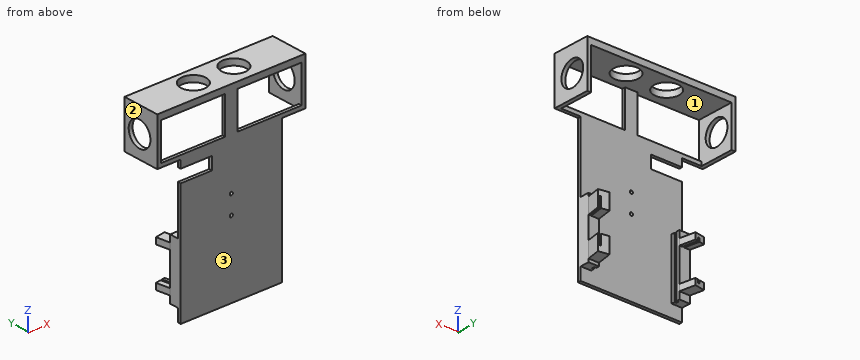
```python
from build123d import *

# Parameters (mm, degrees)
SKETCH1_W            = 95
SKETCH1_H            = 22
SKETCH1_R            = 8
BOSS_EXTRUDE1_DEPTH  = 4
SKETCH2_W            = 41
SKETCH2_H            = 23.5
BOSS_EXTRUDE2_DEPTH  = 2
BOSS_EXTRUDE3_START  = -70
BOSS_EXTRUDE3_DEPTH  = 38
BOSS_EXTRUDE5_DEPTH  = 10
BOSS_EXTRUDE6_DEPTH  = 10
SKETCH10_R           = 1
CUT_EXTRUDE1_DEPTH   = 4
BOSS_EXTRUDE11_START = 45
SKETCH11_W           = 30
SKETCH11_H           = 24
SKETCH11_R           = 8
BOSS_EXTRUDE11_DEPTH = 2.5
BOSS_EXTRUDE12_START = -47.5
SKETCH11_2_W         = 30
SKETCH11_2_H         = 24
SKETCH11_2_R         = 8
BOSS_EXTRUDE12_DEPTH = 2.5


with BuildPart() as part:
    # Sketch1 → Boss-Extrude1 (new body)
    with BuildSketch(Plane.XY):
        Rectangle(SKETCH1_W, SKETCH1_H)
        with Locations((-13, 0)):
            Circle(SKETCH1_R, mode=Mode.SUBTRACT)
        with Locations((13, 0)):
            Circle(SKETCH1_R, mode=Mode.SUBTRACT)
    extrude(amount=BOSS_EXTRUDE1_DEPTH)

    # Sketch2 → Boss-Extrude2 (add)
    with BuildSketch(Plane(origin=(0, -11, 0), x_dir=(-1, 0, 0), z_dir=(0, -1, 0))):
        Polygon((-32.5, 116), (32.5, 116), (32.5, 39), (12.5, 39), (12.5, 31), (32.5, 31), (32.5, 26), (47.5, 26), (47.5, -4), (32.5, -4), (-32.5, -4), (-47.5, -4), (-47.5, 26), (-32.5, 26), align=None)
        with Locations((-24.5, 11.75)):
            Rectangle(SKETCH2_W, SKETCH2_H, mode=Mode.SUBTRACT)
        with Locations((24.5, 11.75)):
            Rectangle(SKETCH2_W, SKETCH2_H, mode=Mode.SUBTRACT)
    extrude(amount=BOSS_EXTRUDE2_DEPTH)

    # Sketch4 → Boss-Extrude3 (add)
    with BuildSketch(Plane.XY.offset(BOSS_EXTRUDE3_START)):
        Polygon((-25.8, -11), (-25.8, -9), (-27, -9), (-27, -7.3), (-25.8, -7.3), (-25.8, -5.3), (-32.5, -5.3), (-32.5, -11), align=None)
        Polygon((32.5, -5.3), (32.5, -11), (25.8, -11), (25.8, -9), (27, -9), (27, -7.3), (25.8, -7.3), (25.8, -5.3), align=None)
    extrude(amount=-BOSS_EXTRUDE3_DEPTH)

    # Sketch7 → Boss-Extrude5 (add)
    with BuildSketch(Plane(origin=(0.128388188, -0.728125596, 0), x_dir=(0, 0, 1), z_dir=(-0.17364817766693402, 0.9848077530122075, 0))):
        Polygon((-74.5, -26.328375369), (-74.5, -32.926587315), (-78.5, -32.926587315), (-78.5, -29.426587315), (-76.5, -29.426587315), (-76.5, -28.226587315), (-78.5, -28.226587315), (-78.5, -26.328375369), align=None)
        Polygon((-101.5, -28.226587315), (-99.5, -28.226587315), (-99.5, -26.328375369), (-103.5, -26.328375369), (-103.5, -32.926587315), (-99.5, -32.926587315), (-99.5, -29.426587315), (-101.5, -29.426587315), align=None)
    extrude(amount=BOSS_EXTRUDE5_DEPTH)

    # Sketch8 → Boss-Extrude6 (add)
    with BuildSketch(Plane(origin=(-0.128388188, -0.728125596, 0), x_dir=(0, 0, 1), z_dir=(0.17364817766692736, 0.9848077530122086, 0))):
        Polygon((-82, 26.328375369), (-82, 31.176587315), (-75.5, 31.176587315), (-75.5, 32.226587315), (-82, 32.226587315), (-82, 32.926587315), (-72, 32.926587315), (-72, 26.328375369), align=None)
        Polygon((-96, 32.226587315), (-96, 32.926587315), (-106, 32.926587315), (-106, 26.328375369), (-96, 26.328375369), (-96, 31.176587315), (-102.5, 31.176587315), (-102.5, 32.226587315), align=None)
    extrude(amount=BOSS_EXTRUDE6_DEPTH)

    # Sketch10 → Cut-Extrude1 (cut)
    with BuildSketch(Plane.XZ.offset(13)):
        with Locations((0, -56)):
            Circle(SKETCH10_R)
        with Locations((0, -68)):
            Circle(SKETCH10_R)
    extrude(amount=-CUT_EXTRUDE1_DEPTH, mode=Mode.SUBTRACT)

    # Sketch11 → Boss-Extrude11 (add)
    with BuildSketch(Plane(origin=(0, 0, 0), x_dir=(0, 0, -1), z_dir=(1, 0, 0)).offset(BOSS_EXTRUDE11_START)):
        with Locations((11, -1)):
            Rectangle(SKETCH11_W, SKETCH11_H)
        with Locations((12, 0)):
            Circle(SKETCH11_R, mode=Mode.SUBTRACT)
    extrude(amount=BOSS_EXTRUDE11_DEPTH)

    # Sketch11<2> → Boss-Extrude12 (add)
    with BuildSketch(Plane(origin=(0, 0, 0), x_dir=(0, 0, -1), z_dir=(1, 0, 0)).offset(BOSS_EXTRUDE12_START)):
        with Locations((11, -1)):
            Rectangle(SKETCH11_2_W, SKETCH11_2_H)
        with Locations((12, 0)):
            Circle(SKETCH11_2_R, mode=Mode.SUBTRACT)
    extrude(amount=BOSS_EXTRUDE12_DEPTH)


solid = part.part
```
Source: CAD feature listing. Evaluate the final solid. Frame: model axes, mm. Face numbers are marked on the shaded views. Give positions to 0.01 mm unless a question says otherwise; leave off trailing zeros. Loops run counter-clockwise (first coordinate to the right, second up) from the corner with the lowest first, then second, coordinate; pieces in that order, holes last. Notation, with made-up numbers: (72, -32.75) - (78, -32.75) arc R35 cw to (78, 2.25) - close; hole circle Ø3 at (84, -18). An arc over 180 degrees is marked (long way). Use CSV: the item, a comma, the result in double quotes. Start each with the question number.
1. Draft query along X for the marked faces 1, 2 and 3. Return one class per face: +X half, -X half, draft (parallel to the pull), parting line (faces both ways), or undercut.
2. Ray query, L1, parallel to X at y = -11.65, z = -68; L2, parallel to X at y = -6, z = -24; L3, parallel to Y at x = 46, z = -12. Return the intervals inside material, ascending.
3. Section C-C (x = 23). Output: boundary loops of the cut face in (y, z).
4. Section B-B (z = -17). Output: boundary loops of the cut face in (x, y) (3 decimals), then the cut area to 4 significant figures.
5. Section A-A (x = 13). Output: boundary loops of the cut face in (y, z), then the cut area to 3 significant figures.
6. Section D-D (z = -91.5). Output: boundary loops of the cut face in (x, y).
7. Pin query (flat end, axial travel): pin 1 (6 mm diameter, centred on y = -8, z = -85.5, fed in from -X); pin 2 (1 mm diameter, centred on x = -26, z = -83, fed in from +Y); pin 3 (12 mm diameter, centred on y = -7, z = -35, fed in from +X); pin 4 (12 mm diameter, centred on y = -6.5, z = -15.5, fed in from -X). Return the tip coordinate at first contact, or that it passes through.
Response:
1,face 1,"undercut"
1,face 2,"-X half"
1,face 3,"draft"
2,L1,"-32.5 to -1, 1 to 32.5"
2,L2,"-47.5 to -45, 45 to 47.5"
2,L3,"-13 to -8, 8 to 11"
3,outline,"(-13, -116) - (-11, -116) - (-11, -23.5) - (-13, -23.5) - close; (-13, 0) - (11, 0) - (11, 4) - (-13, 4) - close"
4,outline,"(-47.5, -13) - (-45, -13) - (-45, -6.245) - (-47.5, -6.245) - close; (-47.5, 6.245) - (-45, 6.245) - (-45, 11) - (-47.5, 11) - close; (-4, -13) - (4, -13) - (4, -11) - (-4, -11) - close; (45, -13) - (47.5, -13) - (47.5, -6.245) - (45, -6.245) - close; (45, 6.245) - (47.5, 6.245) - (47.5, 11) - (45, 11) - close"
4,area,"73.55 mm²"
5,outline,"(-13, -116) - (-11, -116) - (-11, -23.5) - (-13, -23.5) - close; (-13, 0) - (-8, 0) - (-8, 4) - (-13, 4) - close; (8, 0) - (11, 0) - (11, 4) - (8, 4) - close"
5,area,"217 mm²"
6,outline,"(-32.5, -13) - (32.5, -13) - (32.5, -5.3) - (25.8, -5.3) - (25.8, -7.3) - (27, -7.3) - (27, -9) - (25.8, -9) - (25.8, -11) - (-25.8, -11) - (-25.8, -9) - (-27, -9) - (-27, -7.3) - (-25.8, -7.3) - (-25.8, -5.3) - (-32.5, -5.3) - close"
7,pin 1,"x = -32.5"
7,pin 2,"y = -5.3"
7,pin 3,"x = 32.5"
7,pin 4,"x = -47.5"
